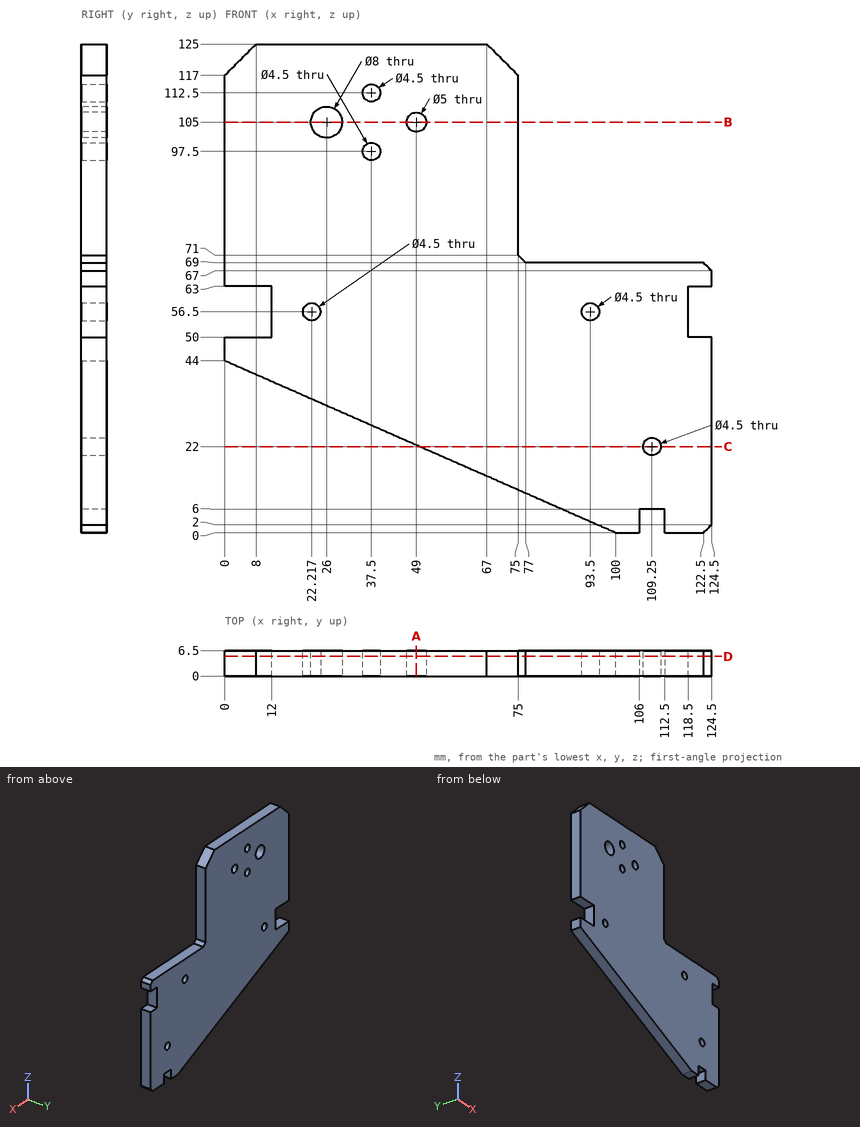
Print and shaded views of the part. All mm, measured from the part's lowest x, y and z. Give positions to 0.01 mm unless a question says otherwise; leave off trailing zeros. Order: outer loops, then holes, each group sorted by start corner. A loop starts at its lowest first (then second) coordinate and runs counter-clockwise, first axis right, second up. Notation, with made-up numbers: (54.5, -11.5) - (87.5, -11.5) arc R29 cw to (87.5, 19.5) - close; hole circle Ø2 at (40, 33.5). An arc over 180 degrees is marked (long way). Use a Markdown table: item, result.
1) Probe L1, parallel to Z at x = 119.5, y = 6; L2, parallel to Z at x = 37.5, y = 4.5; L3, parallel to Z at x = 36, y = 1. List the from-to ranges inside material, lowest first. Write a range as from..to.
Checked values:
| item | result |
|---|---|
| L1 | 0..50, 63..69 |
| L2 | 27.5..95.25, 99.75..110.25, 114.75..125 |
| L3 | 28.16..95.82, 99.18..110.82, 114.18..125 |
2) Saw through at A-A on x = 49. List the corners of the cut face in (y, z).
Checked values:
| item | result |
|---|---|
| outline | (0, 22.44) - (6.5, 22.44) - (6.5, 102.5) - (0, 102.5) - close; (0, 107.5) - (6.5, 107.5) - (6.5, 125) - (0, 125) - close |
3) Saw through at B-B on z = 105. List the corners of the cut face in (x, y), plus the area to 3 significant figures.
Checked values:
| item | result |
|---|---|
| outline | (0, 0) - (22, 0) - (22, 6.5) - (0, 6.5) - close; (30, 0) - (46.5, 0) - (46.5, 6.5) - (30, 6.5) - close; (51.5, 0) - (75, 0) - (75, 6.5) - (51.5, 6.5) - close |
| area | 403 mm² |
4) Saw through at D-D on y = 5. Count the separate pieces of the cut face and the enclosed holes in it, plus the area to 3 significant figures.
Checked values:
| item | result |
|---|---|
| separate pieces | 1 |
| enclosed holes | 7 |
| area | 10,100 mm² |
5) Saw through at C-C on z = 22. List the corners of the cut face in (x, y), plus the area to 3 significant figures.
Checked values:
| item | result |
|---|---|
| outline | (50, 0) - (107, 0) - (107, 6.5) - (50, 6.5) - close; (111.5, 0) - (124.5, 0) - (124.5, 6.5) - (111.5, 6.5) - close |
| area | 455 mm² |
6) Flat gauge pins, fed straight in: P1, Ø3, axis at x = 108.5, y = 2, coming from the -Z side; P2, Ø2.5, axis at x = 22.217, z = 56.5, coming from the +Y side; P3, Ø2, axis at x = 5.5, y = 4, coming from the +Z side; P4, Ø2, axis at y = 3, z = 54, coming from the -X side. Where does each tip first touch, or does it go through?
Checked values:
| item | result |
|---|---|
| P1 | z = 6 |
| P2 | through |
| P3 | z = 123.5 |
| P4 | x = 12 |
